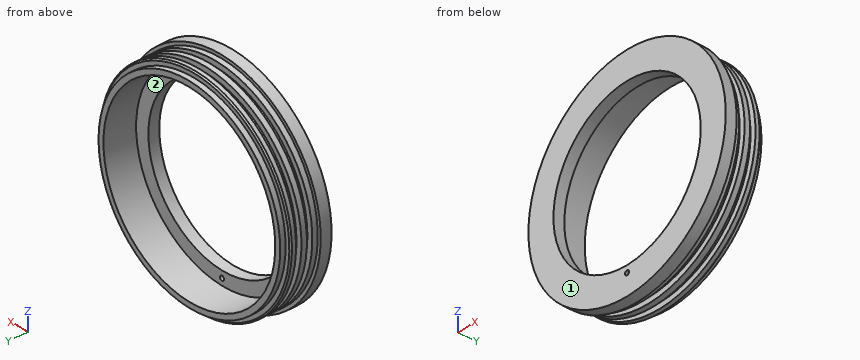
```python
from build123d import *

# Parameters (mm, degrees)
SKETCH1_R           = 51.054
SKETCH1_R_2         = 38.1
BOSS_EXTRUDE1_DEPTH = 5.08
SKETCH2_R           = 49.53
SKETCH2_R_2         = 44.45
BOSS_EXTRUDE2_DEPTH = 15.24
SKETCH4_W           = 2.54
SKETCH4_H           = 2.54
CHAMFER1_SIZE       = 0.635
CUT_EXTRUDE1_DEPTH  = 26.67


with BuildPart() as part:
    # Sketch1 → Boss-Extrude1 (new body)
    with BuildSketch(Plane(origin=(0, 0, 0), x_dir=(1, 0, 0), z_dir=(0, 1, 0))):
        with Locations(Location((0, 0, 0), (0, 0, 270))):
            Circle(SKETCH1_R)
        with Locations(Location((0, 0, 0), (0, 0, 270))):
            Circle(SKETCH1_R_2, mode=Mode.SUBTRACT)
    extrude(amount=BOSS_EXTRUDE1_DEPTH)

    # Sketch2 → Boss-Extrude2 (add)
    with BuildSketch(Plane(origin=(0, 5.08, 0), x_dir=(1, 0, 0), z_dir=(0, 1, 0))):
        with Locations(Location((0, 0, 0), (0, 0, 90))):
            Circle(SKETCH2_R)
        with Locations(Location((0, 0, 0), (0, 0, 90))):
            Circle(SKETCH2_R_2, mode=Mode.SUBTRACT)
    extrude(amount=BOSS_EXTRUDE2_DEPTH)

    # Sketch4 → Cut-Revolve1 (revolve, cut)
    with BuildSketch(Plane.XY, mode=Mode.PRIVATE) as cut_revolve1_sk:
        with Locations((-48.26, 8.89)):
            Rectangle(SKETCH4_W, SKETCH4_H)
        with Locations((-48.26, 13.97)):
            Rectangle(SKETCH4_W, SKETCH4_H)
        with Locations((-48.26, 19.05)):
            Rectangle(SKETCH4_W, SKETCH4_H)
    revolve(cut_revolve1_sk.sketch.rotate(Axis((0, 0, 0), (0, 1, 0)), 270), axis=Axis((0, 0, 0), (0, 1, 0)), mode=Mode.SUBTRACT)

    # Chamfer1
    chamfer1_edges = [part.edges().sort_by_distance(p)[0] for p in [
        (0, 17.78, 49.53),
    ]]
    chamfer(chamfer1_edges, length=CHAMFER1_SIZE)

    # Sketch5 → Cut-Extrude1 (cut)
    with BuildSketch(Plane(origin=(0, 5.08, 0), x_dir=(1, 0, 0), z_dir=(0, 1, 0))):
        with BuildLine():
            ThreePointArc((0, 42.333333164), (-1.058333164, 41.275), (0, 40.216666836))
            Line((0, 40.216666836), (0, 42.333333164))
        make_face()
        with BuildLine():
            Line((0, 42.333333164), (0, 40.216666836))
            ThreePointArc((0, 40.216666836), (0.748354557, 40.526645443), (1.058333164, 41.275))
            ThreePointArc((1.058333164, 41.275), (0.748354557, 42.023354557), (0, 42.333333164))
        make_face()
    extrude(amount=-CUT_EXTRUDE1_DEPTH, mode=Mode.SUBTRACT)


solid = part.part
```
The model under review builds one solid part; all positions refer to its coordinate system, in mm. Face numbers are marked on the shaded views. Round coordinates to 2 decimals unless told otherwise and drop trailing zeros. Use CSV: the item, a comma, the result in double quotes. Start each with the question number.
(1) Clearance check with flat-ended pins moving along their axes: P1, Ø4, axis at x = -1.5, y = 17, coming from the +Z side; P2, Ø12, axis at x = -12, y = 4, coming from the -Z side; P3, Ø5, axis at y = 14, z = 6.5, coming from the -X side. State where each tip first meets the part, or that it passes through.
(2) For line 1 along Y through (x, z) = (28, 40); line 2 along X through (y, z) = (12.5, 0); line 3 along X through (y, z) = (4, 0), list the stretches that pass through material, from the lowest coordinate up.
(3) The part is to be moulded in two halves that separate along Z. For the marked faces 1 and 2, say which applies: +Z half, -Z half, draft (parallel to the pull), parting line (faces both ways), or undercut.
Findings:
1,P1,"z = 49.53"
1,P2,"z = -50.7"
1,P3,"x = -49.34"
2,line 1,"0 to 7.62, 10.16 to 12.7, 15.24 to 17.78"
2,line 2,"-49.53 to -44.45, 44.45 to 49.53"
2,line 3,"-51.05 to -38.1, 38.1 to 51.05"
3,face 1,"draft"
3,face 2,"undercut"
